Geometry: final body of the model. Coordinates: model frame, mm. A direction names the side the tool comes from. Give positions to 0.01 mm unless a question says otherwise; leave off trailing zeros. Loops run counter-clockwise (first coordinate to the right, second up) from the corner with the lowest first, then second, coordinate; pieces in that order, holes last. Notation, with made-up numbers: M -18,-23 L -5,-23 A22 cw -5,-15 Z; hole C 71.5,69 d9. An arc over 180 degrees is marked long. Put each result on its own line as item: value.
```python
from build123d import *

# Parameters (mm, degrees)
SKETCH_1_R      = 1.55
EXTRUDE_1_DEPTH = 4
FILLET_1_R      = 2


with BuildPart() as part:
    # 草图1 → 凸台-拉伸1 (new body)
    with BuildSketch(Plane(origin=(0, 0, 0), x_dir=(0, 0, -1), z_dir=(1, 0, 0))):
        with BuildLine():
            ThreePointArc((8, 0), (5.656854249, 5.656854249), (0, 8))
            Line((0, 8), (-8, 8))
            Line((-8, 8), (-8, 0))
            Line((-8, 0), (0, 0))
            Line((0, 0), (0, -118.02))
            Line((0, -118.02), (-8, -118.02))
            Line((-8, -118.02), (-8, -126.02))
            Line((-8, -126.02), (0, -126.02))
            ThreePointArc((0, -126.02), (5.656854249, -123.676854249), (8, -118.02))
            Line((8, -118.02), (8, 0))
        make_face()
        with Locations((-4, 4)):
            Circle(SKETCH_1_R, mode=Mode.SUBTRACT)
        with Locations((-4, -122.02)):
            Circle(SKETCH_1_R, mode=Mode.SUBTRACT)
    extrude(amount=EXTRUDE_1_DEPTH)

    # 圆角1
    fillet_1_edges = [part.edges().sort_by_distance(p)[0] for p in [
        (2, -126.02, 8),
        (2, -118.02, 8),
        (2, -118.02, 0),
        (2, 0, 0),
        (2, 0, 8),
        (2, 8, 8),
    ]]
    fillet(fillet_1_edges, radius=FILLET_1_R)


solid = part.part
```
Item 1: Section D-D on y = -34. Output: boundary loops of the cut face in (x, z).
Output values:
outline: M 0,-8 L 4,-8 L 4,0 L 0,0 Z
Item 2: Mould query, pull axis Z, two halves, no side actions, for faces 1 (the cylindrical face through (2, -123, 5.2)), 2 (the cylindrical face through (1.972, -123.739, -5.594)), 3 (the cylindrical face through (1.97, 4.07, 5.55)), 4 (the flat face through (2, -118.02, 4)). Classes: pulls with the +Z half, pulls with the -Z half, needs draft (parallel to the pull), parting line crosses it, or undercut.
Output values:
face 1: undercut
face 2: pulls with the -Z half
face 3: undercut
face 4: needs draft
Item 3: Pin query (flat end, axial travel): pin 1 Ø1.5 at (y, z) = (-38, -3.5) entering from -X; pin 2 Ø2 at (x, y) = (2.5, -74) entering from +Z. Return the tip coordinate at first contact, or that it passes through.
Output values:
pin 1: x = 0
pin 2: z = 0
Item 4: Section B-B on z = 4. Output: boundary loops of the cut face in (x, y), then the cut area to 3 significant figures.
Output values:
outline: M 0,-126.02 L 4,-126.02 L 4,-123.57 L 0,-123.57 Z; M 0,-120.47 L 4,-120.47 L 4,-118.02 L 0,-118.02 Z; M 0,0 L 4,0 L 4,2.45 L 0,2.45 Z; M 0,5.55 L 4,5.55 L 4,8 L 0,8 Z
area: 39.2 mm²
Item 5: Section C-C on y = 4. Output: boundary loops of the cut face in (x, z).
Output values:
outline: M 0,-6.93 L 4,-6.93 L 4,2.45 L 0,2.45 Z; M 0,5.55 L 4,5.55 L 4,8 L 0,8 Z
Item 6: Set-up query: faces 5 (the flat face through (2, -122, 8)), 6 (the flat face through (2, 0, 4)). Return all of +Z, -Z, +X, -X, +Y, -Y with unobstructed straight access to the full face (end or side cutting, diameter ignored); none if empty.
Output values:
face 5: +Z, +X, -X, +Y, -Y
face 6: +Z, +X, -X
Item 7: Section A-A on x = 0.8. Output: boundary loops of the cut face in (y, z).
Output values:
outline: M -126.02,0 A8 ccw -118.02,-8 L 0,-8 A8 ccw 8,0 L 8,6 A2 ccw 6,8 L 2,8 A2 ccw 0,6 L 0,2 A2 cw -2,0 L -116.02,0 A2 cw -118.02,2 L -118.02,6 A2 ccw -120.02,8 L -124.02,8 A2 ccw -126.02,6 Z; hole C -122.02,4 d3.1; hole C 4,4 d3.1
Item 8: Line query: probe 1 along Y at (x, z) = (1.2, 4); probe 2 along Z at (x, y) = (1.8, -101); probe 3 along Y at (x, z) = (0.5, 2.25). Output: solid intervals per line, ascending. Write a range as [from, to].
Output values:
probe 1: [-126.02, -123.57], [-120.47, -118.02], [0, 2.45], [5.55, 8]
probe 2: [-8, 0]
probe 3: [-126.02, -118.02], [0, 8]
